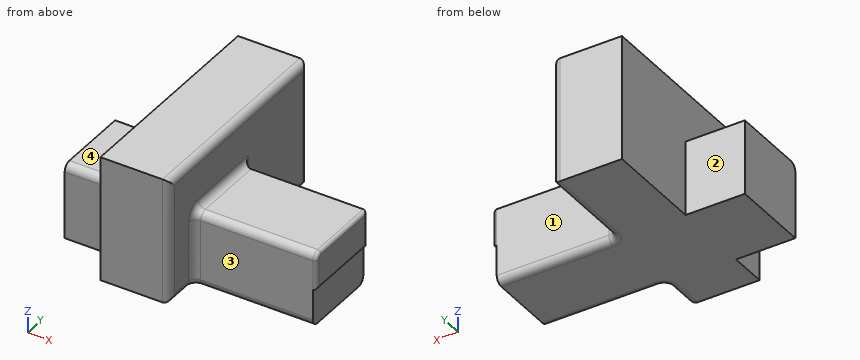
```python
from build123d import *

# Parameters (mm, degrees)
F0_W     = 173.5329478979
F0_H     = 54.4529519975
F1_DEPTH = 25.4
F2_R     = 5.08
F3_R     = 2.54
F4_W     = 47.7339737117
F4_H     = 148.616027087
F5_DEPTH = 60.198
F6_DEPTH = 26.162
F7_R     = 5.08


with BuildPart() as f1:
    # F0 (on Top) → F1 (new body)
    with BuildSketch(Plane.XY):
        with Locations((45.8968058228, 4.7943573445)):
            Rectangle(F0_W, F0_H)
    extrude(amount=F1_DEPTH)

    # F2
    f2_edges = [f1.edges().sort_by_distance(p)[0] for p in [
        (45.896806, -22.432119, 25.4),
    ]]
    fillet(f2_edges, radius=F2_R)

    # F3
    f3_edges = [f1.edges().sort_by_distance(p)[0] for p in [
        (132.66328, -22.432119, 10.16),
        (132.66328, -20.944221, 23.912102),
        (132.66328, 4.794357, 0),
        (132.66328, 7.334357, 25.4),
        (132.66328, 32.020833, 12.7),
    ]]
    fillet(f3_edges, radius=F3_R)

    # F4 (on Top) → F5 (join)
    with BuildSketch(Plane.XY):
        with Locations((23.8669868559, 26.4220479876)):
            Rectangle(F4_W, F4_H)
    extrude(amount=F5_DEPTH)

    # F6 (add): a face of the model
    f6_faces = [f1.faces().sort_by_distance(p)[0] for p in [
        (37.8680200683, 15.9075868005, 0),
    ]]
    extrude(f6_faces, amount=F6_DEPTH)

    # F7
    f7_edges = [f1.edges().sort_by_distance(p)[0] for p in [
        (47.733974, -47.885966, 17.018),
        (47.733974, -35.159042, -26.162),
        (47.733974, -22.432119, -2.921),
        (47.733974, -20.944221, 23.912102),
        (47.733974, 7.334357, 25.4),
        (47.733974, 32.020833, -0.381),
        (47.733974, 66.375447, -26.162),
        (47.733974, 100.730062, 17.018),
        (47.733974, 26.422048, 60.198),
        (88.928627, -22.432119, -26.162),
        (88.928627, 32.020833, -26.162),
    ]]
    fillet(f7_edges, radius=F7_R)


solid = f1.part
```
Can you work these out from the model? Positions are in its coordinate system, mm. Face numbers are marked on the shaded views. A direction names the side the tool comes from. Coordinates: 2 decimals unless noted, no trailing zeros. Order: outer loops, then holes, each group sorted by start corner. A loop starts at its lowest first (then second) coordinate and runs counter-clockwise, first axis right, second up.
1. I need wall thicknesses on line 1 (X direction, y = 41.5, z = 23); line 2 (Y direction, x = 69, z = -1); line 3 (X direction, y = -19.5, z = -12.5). Which ranges of each line are inside material? Lowest first, please.
2. I'm going to push flat-ended pins straight in: pin 1 (20.5 mm diameter, centred on x = 85, z = -6, fed in from -Y); pin 2 (24.5 mm diameter, centred on x = 79.5, y = 5.5, fed in from +Z); pin 3 (8 mm diameter, centred on y = 84.5, z = 40.5, fed in from -X). Where does each tip first touch, or does it pass through?
3. If we section it at A-A (x = 95.5): Please give me the cut outline in (y, z), then the cut area to 3 significant figures.
4. For the marked faces 1, 2, 3 and 4, which set-ups out of +Z, -Z, +X, -X, +Y, -Y let a thin tool reach every point of the face, with its end or its side?
5. If we section it at B-B (z = -17.5): Please give me the cut outline in (x, y), then the cut area to 3 significant figures.
6. If we section it at D-D (z = 5.5): Please give me the cut outline in (x, y).
7. If we section it at C-C (y = -14.5): Please give me the cut outline in (x, z), then the cut area to 3 significant figures.
Entries:
1. line 1: x = 0 to 47.73
1. line 2: y = -22.43 to 32.02
1. line 3: x = -40.87 to 130.12
2. pin 1: stops at y = -22.43
2. pin 2: stops at z = 25.4
2. pin 3: stops at x = 0
3. outline: (-22.43, -21.08) arc R5.08 ccw to (-17.35, -26.16) - (26.94, -26.16) arc R5.08 ccw to (32.02, -21.08) - (32.02, 25.4) - (-17.35, 25.4) arc R5.08 ccw to (-22.43, 20.32) - close
3. area: 2,790 mm2
4. face 1: +Z, -Z, +X, +Y
4. face 2: +Z, -Z, -X, +Y
4. face 3: +Z, -Z, +X, -Y
4. face 4: +Z, -X, +Y, -Y
5. outline: (-40.87, -22.43) - (0, -22.43) - (0, -47.89) - (42.65, -47.89) arc R5.08 ccw to (47.73, -42.81) - (47.73, -27.51) arc R5.08 cw to (52.81, -22.43) - (130.12, -22.43) - (130.12, 32.02) - (52.81, 32.02) arc R5.08 cw to (47.73, 37.1) - (47.73, 95.65) arc R5.08 ccw to (42.65, 100.73) - (0, 100.73) - (0, 32.02) - (-40.87, 32.02) - close
5. area: 13,800 mm2
6. outline: (-40.87, -22.43) - (0, -22.43) - (0, -47.89) - (42.65, -47.89) arc R5.08 ccw to (47.73, -42.81) - (47.73, -27.51) arc R5.08 cw to (52.81, -22.43) - (130.12, -22.43) arc R2.54 ccw to (132.66, -19.89) - (132.66, 29.48) arc R2.54 ccw to (130.12, 32.02) - (52.81, 32.02) arc R5.08 cw to (47.73, 37.1) - (47.73, 95.65) arc R5.08 ccw to (42.65, 100.73) - (0, 100.73) - (0, 32.02) - (-40.87, 32.02) - close
7. outline: (-40.87, -26.16) - (130.12, -26.16) - (130.12, 0) arc R2.54 ccw to (132.66, 2.54) - (132.66, 22.86) arc R2.54 ccw to (130.12, 25.4) - (52.81, 25.4) arc R5.08 cw to (47.73, 30.48) - (47.73, 55.12) arc R5.08 ccw to (42.65, 60.2) - (0, 60.2) - (0, 25.4) - (-40.87, 25.4) - close
7. area: 10,500 mm2
